Design review of the part shown in the three views and the two pictorial views. Dimensions are in mm from the part's minimum x, y and z. Coordinates: 2 decimals unless noted, no trailing zeros. Loops run counter-clockwise (first coordinate to the right, second up) from the corner with the lowest first, then second, coordinate; pieces in that order, holes last. Notation, with made-up numbers: (2, -33) -> (28, -33) arc R23 ccw to (28, -10) -> close; hole circle Ø11 at (12.5, 52.5). An arc over 180 degrees is marked (long way). One line per item, written item: value.
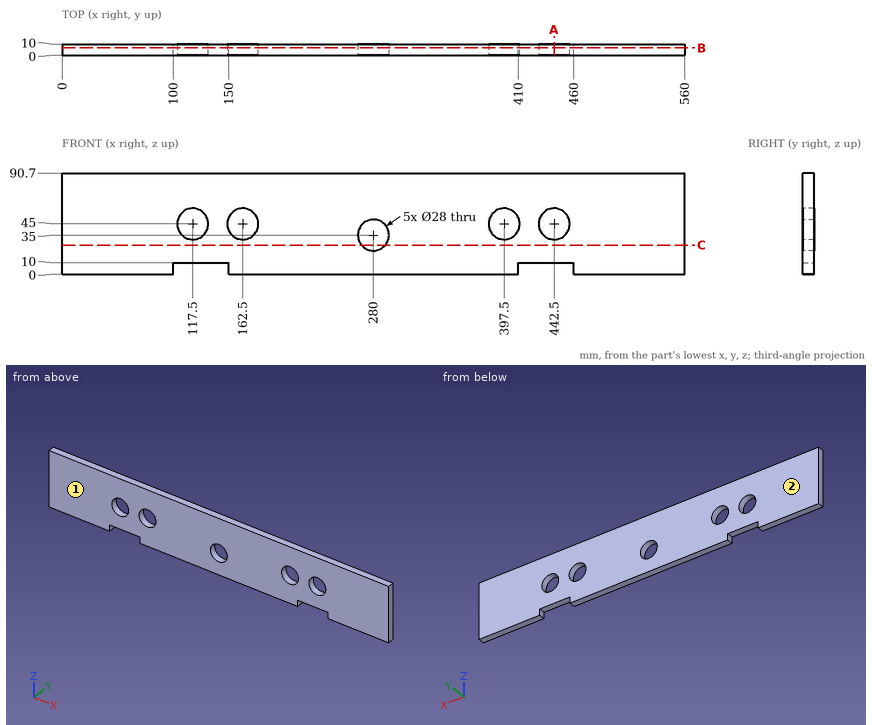
1. Insertion check: pin 1 Ø3 at (x, y) = (120.5, 3) entering from -Z. The pin has a flat end and moves straight along its axis. Give the tip position at first contact, or say it passes through.
Return value:
pin 1: stops at z = 10
2. Take a section at C-C, the plane z = 26. Give the boundary of the cut face in (x, y), and give its area (3 significant figures).
Return value:
outline: (0, 0) -> (269.28, 0) -> (269.28, 10) -> (0, 10) -> close; (290.72, 0) -> (560, 0) -> (560, 10) -> (290.72, 10) -> close
area: 5,390 mm2
3. To check wall thickness, follow probe 1 along X at (y, z) = (4, 6); probe 2 along Z at (x, y) = (442.5, 3.75); probe 3 along Z at (x, y) = (397.5, 7.25). State the ranges of each line that lie inside material, in increasing order. Write a range as from..to.
Return value:
probe 1: x = 0..100, 150..410, 460..560
probe 2: z = 10..31, 59..90.7
probe 3: z = 0..31, 59..90.7
4. Take a section at B-B, the plane y = 6.5. Give the boundary of the cut face in (x, z), and give its area (3 significant figures).
Return value:
outline: (0, 0) -> (100, 0) -> (100, 10) -> (150, 10) -> (150, 0) -> (410, 0) -> (410, 10) -> (460, 10) -> (460, 0) -> (560, 0) -> (560, 90.7) -> (0, 90.7) -> close; hole circle Ø28 at (117.5, 45); hole circle Ø28 at (162.5, 45); hole circle Ø28 at (280, 35); hole circle Ø28 at (397.5, 45); hole circle Ø28 at (442.5, 45)
area: 46,700 mm2
5. The part is to be moulded in two halves that separate along Y. For the marked faces 1 and 2, say which applies: pulls with the +Y half, pulls with the -Y half, needs draft (parallel to the pull), parting line crosses it, or undercut.
Return value:
face 1: pulls with the -Y half
face 2: pulls with the +Y half
6. Take a section at A-A, the plane x = 442.5. Give the boundary of the cut face in (y, z), and give its area (3 significant figures).
Return value:
outline: (0, 10) -> (10, 10) -> (10, 31) -> (0, 31) -> close; (0, 59) -> (10, 59) -> (10, 90.7) -> (0, 90.7) -> close
area: 527 mm2
